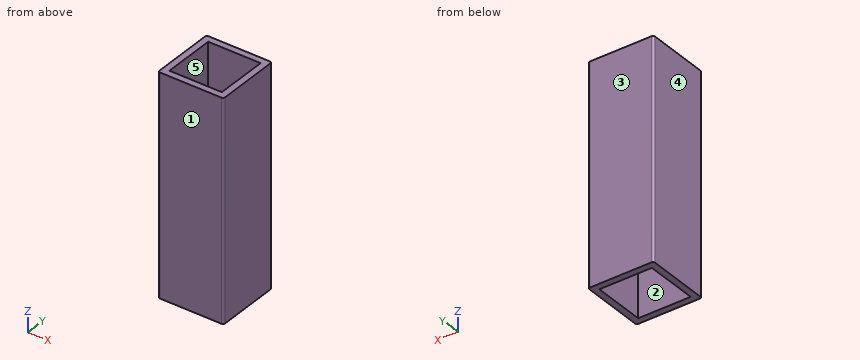
```python
from build123d import *

# Parameters (mm, degrees)
SKETCH_W   = 30
SKETCH_H   = 30
SKETCH_W_2 = 24
SKETCH_H_2 = 24
PAD_DEPTH  = 100
FILLET_R   = 1


with BuildPart() as part:
    # Sketch → Pad (new body)
    with BuildSketch(Plane.XY):
        Rectangle(SKETCH_W, SKETCH_H)
        Rectangle(SKETCH_W_2, SKETCH_H_2, mode=Mode.SUBTRACT)
    extrude(amount=PAD_DEPTH)

    # Fillet
    fillet_edges = [part.edges().sort_by_distance(p)[0] for p in [
        (15, -15, 50),
        (15, 15, 50),
        (-15, -15, 50),
        (-15, 15, 50),
    ]]
    fillet(fillet_edges, radius=FILLET_R)


solid = part.part
```
Source: CAD feature listing. Evaluate the final solid. Frame: model axes, mm. Face numbers are marked on the shaded views. A direction names the side the tool comes from. Coordinates: 2 decimals unless noted, no trailing zeros. Write each loop counter-clockwise with the first axis right and the second up, starting at its lowest first coordinate (ties: lowest second). Pieces come first, ordered by that corner, then holes. Notation, with made-up numbers: (13.5, -25) -> (34.5, -25) arc R21 cw to (34.5, 9) -> close; hole circle Ø8 at (28, -23). An arc over 180 degrees is marked (long way). Return JSON: item names as keys, results as strings. Group by question number.
1) Section query B-B, the plane z = 29.5. Return loops of the section in (x, y).
2) Ray query, line 1 along X through (y, z) = (6.5, 16.5). Return the intervals inside material, ascending.
3) Mould query, pull axis Y, two halves, no side actions, for the marked faces 3, 4 and 5. Classes: +Y half, -Y half, draft (parallel to the pull), parting line (faces both ways), or undercut.
4) Section query A-A, the plane y = -7. Return loops of the section in (x, z), plus the area to 3 significant figures.
5) Set-up query: the marked faces 1 and 2. Return all of +Z, -Z, +X, -X, +Y, -Y with unobstructed straight access to the full face (end or side cutting, diameter ignored); none if empty.
6) Contact query for a flat-ended pin moving along its axis: P1, Ø8, axis at x = 6, y = 11, coming from the +Z side. Output: stop coordinate, or through.
From the geometry:
{
 "1": {"outline": "(-15, -14) arc R1 ccw to (-14, -15) -> (14, -15) arc R1 ccw to (15, -14) -> (15, 14) arc R1 ccw to (14, 15) -> (-14, 15) arc R1 ccw to (-15, 14) -> close; hole (-12, -12) -> (12, -12) -> (12, 12) -> (-12, 12) -> close"},
 "2": {"line 1": "-15 to -12, 12 to 15"},
 "3": {"face 3": "+Y half", "face 4": "draft", "face 5": "undercut"},
 "4": {"outline": "(-15, 0) -> (-12, 0) -> (-12, 100) -> (-15, 100) -> close; (12, 0) -> (15, 0) -> (15, 100) -> (12, 100) -> close", "area": "600 mm²"},
 "5": {"face 1": "+Z, -Z, +X, -X, -Y", "face 2": "+Z, -Z"},
 "6": {"P1": "z = 100"}
}
